Input: part model. Units: mm. Frame: model coordinates. Face numbers are marked on the shaded views. A direction names the side the tool comes from. Round coordinates to 2 decimals unless told otherwise and drop trailing zeros. Write each loop counter-clockwise with the first axis right and the second up, starting at its lowest first coordinate (ties: lowest second). Pieces come first, ordered by that corner, then holes. Notation, with made-up numbers: (73.5, 16.25) -> (77.5, 16.25) arc R33 cw to (77.5, 49.25) -> close; hole circle Ø8 at (79.25, 45.25). An arc over 180 degrees is marked (long way). Write item = value, one per line.
Autodesk Inventor part; units mm, degrees
ref_plane "YZ Plane" through (0, 0, 0) normal (1, 0, 0) x (0, 1, 0)
ref_plane "XZ Plane" through (0, 0, 0) normal (0, 1, 0) x (-1, 0, 0)
ref_plane "XY Plane" through (0, 0, 0) normal (0, 0, 1) x (1, 0, 0)
sketch "Sketch1" plane through (0, 0, 0) normal (0, 1, 0) x (-1, 0, 0)
  line L0 (0.9994, -10) -> (3.0006, -10)
  ellipse E0 centre (2.9994, -8.9994) end of major axis (3.7074, -9.7074) minor radius 1 (3.0006, -10) -> (4, -9.0006) ccw
  line L1 (4, -9.0006) -> (4, -0.9994)
  ellipse E1 centre (2.9994, -1.0006) end of major axis (3.7074, -0.2926) minor radius 1 (4, -0.9994) -> (3.0006, 0) ccw
  line L2 (3.0006, 0) -> (0.9994, 0)
  ellipse E2 centre (1.0006, -1.0006) end of major axis (1.7086, -1.7086) minor radius 1 (0.9994, 0) -> (0, -0.9994) ccw
  line L3 (0, -0.9994) -> (0, -9.0006)
  ellipse E3 centre (1.0006, -8.9994) end of major axis (1.7086, -8.2914) minor radius 1 (0, -9.0006) -> (0.9994, -10) ccw
  circle A0 centre (2, -5) radius 1.75
  circle A1 centre (2, -5) radius 1.25
  line L4 (0, 0) -> (4, 0)
  line L5 (4, 0) -> (4, -10)
  line L6 (4, -10) -> (0, -10)
  line L7 (0, -10) -> (0, 0)
  circle A2 centre (2, -5) radius 1.05
  point P0 (0, -5)
  dimension "d3" = 1
  dimension "d7" = 1.0013
  dimension "d0" = 2.5
  dimension "d1" = 4
  dimension "d2" = 10
  dimension "d4" = 2
  dimension "d5" = 3.5
  dimension "d13" = 5
  dimension "d20" = 0.2
extrude "Extrusion1" add sketch "Sketch1" along normal blind 2 contours E3 L3 E2 L2 E1 L1 E0 L0 | A0 | A1 | A2
extrude "Extrusion2" add sketch "Sketch1" against normal blind 2.5 contours A2
properties part number "flipper_robot_v1_flipper_adapter"
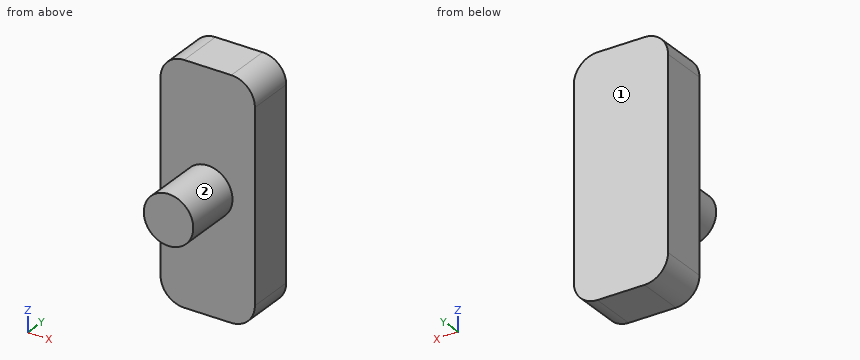
1) Cut plane A-A (z = -5). Return the cut outline in (x, y).
Solutions:
outline = (-4, 0) -> (-3.05, 0) -> (-3.05, -2.5) -> (-0.95, -2.5) -> (-0.95, 0) -> (0, 0) -> (0, 2) -> (-4, 2) -> close
2) First-contact query: P1, Ø2, axis at y = -2, z = -6.5, coming from the +X side. Flat tip, straight axial feed; report the tip coordinate or a pass-through.
Solutions:
P1 = -1.08
3) Cut plane B-B (x = -1.75). Return the cut outline in (y, z), and give its area (3 significant figures).
Solutions:
outline = (-2.5, -6.02) -> (0, -6.02) -> (0, -10) -> (2, -10) -> (2, 0) -> (0, 0) -> (0, -3.98) -> (-2.5, -3.98) -> close
area = 25.1 mm^2
4) Line query: L1, parallel to Y at x = -0.65, z = -3.5; L2, parallel to Z at x = -2.7, y = -1.05; L3, parallel to Z at x = -2.3, y = -1.85. Output: solid intervals per line, ascending. Write a range as from..to.
Solutions:
L1 = 0..2
L2 = -5.78..-4.22
L3 = -6.01..-3.99
5) Cut plane D-D (z = -7.5). Return the cut outline in (x, y).
Solutions:
outline = (-4, 0) -> (0, 0) -> (0, 2) -> (-4, 2) -> close
6) Access query for the marked faces 1 and 2. Directions: +Z, -Z, +X, -X, +Y, -Y. A direction counts if a zero-diameter tool reaches every point of the face in a straight line with its end or side. Return the directions, or none.
Solutions:
face_1 = +Z, -Z, +X, -X, +Y
face_2 = -Y
7) Cut plane C-C (y = -1.8). Return the cut outline in (x, z), and give its area (3 significant figures).
Solutions:
outline = circle Ø2.1 at (-2, -5)
area = 3.46 mm^2
